Autodesk Fusion 360 part; units mm, degrees
sketch "Sketch1" plane through (0, 0, 0) normal (0, 1, 0) x (1, 0, 0)
  line L0 (7, -3.5) -> (-7, -3.5)
  line L1 (-7, -3.5) -> (-7, 3.5)
  line L2 (-7, 3.5) -> (7, 3.5)
  line L3 (7, 3.5) -> (7, -3.5)
  line L4 (7, -3.5) -> (-7, 3.5) construction
  line L5 (-7, -3.5) -> (7, 3.5) construction
  circle A0 centre (-6, 0) radius 0.5
  circle A1 centre (-1, 0) radius 0.5
  circle A2 centre (1, 0) radius 0.5
  circle A3 centre (6, 0) radius 0.5
  dimension "d3" = 14
  dimension "d4" = 7
  dimension "d7" = 1
  dimension "d8" = 1
  dimension "d9" = 1
  dimension "d10" = 1
sketch "Sketch2" plane through (0, 0, 0) normal (0, -1, 0) x (1, 0, 0)
  circle A0 centre (-1, 0) radius 0.5
  circle A1 centre (1, 0) radius 0.5
  circle A2 centre (6, 0) radius 0.5
  circle A3 centre (-6, 0) radius 0.5
  line L0 (-7, -3.5) -> (7, -3.5)
  line L1 (7, -3.5) -> (7, 3.5)
  line L2 (7, 3.5) -> (-7, 3.5)
  line L3 (-7, 3.5) -> (-7, -3.5)
  line L4 (-6, 2.5) -> (-6, -2.5)
  line L5 (6, -2.5) -> (6, 2.5)
  line L6 (6, -2.5) -> (1, -2.5)
  line L7 (1, -2.5) -> (1, 2.5)
  line L8 (1, 2.5) -> (6, 2.5)
  line L9 (-6, -2.5) -> (-6, 2.5)
  line L10 (-6, 2.5) -> (-1, 2.5)
  line L11 (-1, 2.5) -> (-1, -2.5)
  line L12 (-1, -2.5) -> (-6, -2.5)
sketch "Sketch3" plane through (0, 0, 0) normal (0, -1, 0) x (1, 0, 0)
sketch "Sketch4" plane through (0, 0, 0) normal (0, 1, 0) x (1, 0, 0)
  line L0 (-8, -5) -> (8, -5)
  line L1 (8, -5) -> (8, 5)
  line L2 (8, 5) -> (-8, 5)
  line L3 (-8, 5) -> (-8, -5)
  line L4 (-8, -5) -> (8, 5) construction
  line L5 (8, -5) -> (-8, 5) construction
  line L6 (-1, 0) -> (-1, -3)
  line L7 (-1, -3) -> (-7, -3)
  line L8 (-7, -3) -> (-7, 3)
  line L9 (-7, 3) -> (-1, 3)
  line L10 (-1, 3) -> (-1, 0)
  line L11 (1, 3) -> (1, -3)
  line L12 (1, -3) -> (7, -3)
  line L13 (7, -3) -> (7, 3)
  line L14 (7, 3) -> (1, 3)
  dimension "d16" = 16
  dimension "d17" = 10
sketch "Sketch5" plane through (0, 0, 0) normal (0, -1, 0) x (1, 0, 0)
  line L0 (-8, 5) -> (-8, -5)
  line L1 (-8, -5) -> (8, -5)
  line L2 (8, -5) -> (8, 5)
  line L3 (8, 5) -> (-8, 5)
  line L4 (-1, -3) -> (-1, 3)
  line L5 (-1, 3) -> (-7, 3)
  line L6 (-7, 3) -> (-7, -3)
  line L7 (-7, -3) -> (-1, -3)
  line L8 (1, -3) -> (1, 3)
  line L9 (1, 3) -> (7, 3)
  line L10 (7, 3) -> (7, -3)
  line L11 (7, -3) -> (1, -3)
sketch "Sketch6" plane through (0, 0, 0) normal (0, -1, 0) x (1, 0, 0)
  line L0 (-1, 3) -> (-1, -3)
  line L1 (-1, -3) -> (-7, -3)
  line L2 (-7, -3) -> (-7, 3)
  line L3 (-7, 3) -> (-1, 3)
  line L4 (1, 3) -> (7, 3)
  line L5 (7, 3) -> (7, -3)
  line L6 (7, -3) -> (1, -3)
  line L7 (1, -3) -> (1, 3)
  line L8 (-8, 5) -> (-8, -5)
  line L9 (-8, -5) -> (8, -5)
  line L10 (8, -5) -> (8, 5)
  line L11 (8, 5) -> (-8, 5)
  circle A0 centre (-7, 0) radius 0.25
  circle A1 centre (-1, 0) radius 0.25
  circle A2 centre (1, 0) radius 0.25
  circle A3 centre (7, 0) radius 0.25
  dimension "d23" = 0.5
  dimension "d24" = 0.5
  dimension "d25" = 0.5
  dimension "d26" = 0.5
sketch "Sketch7" plane through (0, 4, 0) normal (0, 1, 0) x (-1, 0, 0)
  circle A0 centre (1, 0) radius 0.25
  circle A1 centre (-1, 0) radius 0.25
  circle A2 centre (7, 0) radius 0.25
  circle A3 centre (-7, 0) radius 0.25
  line L0 (8, -5) -> (8, 5)
  line L1 (8, 5) -> (-8, 5)
  line L2 (-8, 5) -> (-8, -5)
  line L3 (-8, -5) -> (8, -5)
  line L4 (-10, -7) -> (10, -7)
  line L5 (10, -7) -> (10, 7)
  line L6 (10, 7) -> (-10, 7)
  line L7 (-10, 7) -> (-10, -7)
  circle A4 centre (-7, 0) radius 0.25
  circle A5 centre (-1, 0) radius 0.25
  circle A6 centre (1, 0) radius 0.25
  circle A7 centre (7, 0) radius 0.25
  dimension "d29" = 2
sketch "Sketch8" plane through (0, 0, 0) normal (0, -1, 0) x (1, 0, 0)
  line L0 (-8, 5) -> (-8, -5)
  line L1 (-8, -5) -> (8, -5)
  line L2 (8, -5) -> (8, 5)
  line L3 (8, 5) -> (-8, 5)
  arc A0 (1, 0.25) -> (1, -0.25) centre (1, 0) ccw
  line L4 (1, 0.25) -> (1, 3)
  line L5 (1, 3) -> (7, 3)
  line L6 (7, 3) -> (7, 0.25)
  arc A1 (7, -0.25) -> (7, 0.25) centre (7, 0) ccw
  line L7 (7, -0.25) -> (7, -3)
  line L8 (7, -3) -> (1, -3)
  line L9 (1, -3) -> (1, -0.25)
  arc A2 (-1, -0.25) -> (-1, 0.25) centre (-1, 0) ccw
  line L10 (-1, -0.25) -> (-1, -3)
  line L11 (-1, -3) -> (-7, -3)
  line L12 (-7, -3) -> (-7, -0.25)
  arc A3 (-7, 0.25) -> (-7, -0.25) centre (-7, 0) ccw
  line L13 (-7, 0.25) -> (-7, 3)
  line L14 (-7, 3) -> (-1, 3)
  line L15 (-1, 3) -> (-1, 0.25)
  circle A4 centre (-6.5, 4) radius 0.5
  circle A5 centre (-6.5, -4) radius 0.5
  circle A6 centre (6.5, -4) radius 0.5
  circle A7 centre (6.5, 4) radius 0.5
ref_plane "WorkPlane1" through (0, -6, 0) normal (0, -1, 0) x (-1, 0, 0)
sketch "Sketch11" plane through (0, 0, 0) normal (0, -1, 0) x (1, 0, 0)
sketch "Sketch12" plane through (0, 4, 0) normal (0, 1, 0) x (-1, 0, 0)
  circle A0 centre (1, 0) radius 0.25
  circle A1 centre (-1, 0) radius 0.25
  circle A2 centre (7, 0) radius 0.25
  circle A3 centre (-7, 0) radius 0.25
  line L0 (-11, -8) -> (11, -8)
  line L1 (11, -8) -> (11, 8)
  line L2 (11, 8) -> (-11, 8)
  line L3 (-11, 8) -> (-11, -8)
sketch "Sketch13" plane through (0, 0, 0) normal (0, -1, 0) x (1, 0, 0)
sketch "Sketch14" plane through (0, 0, 0) normal (0, -1, 0) x (1, 0, 0)
sketch "Sketch15" plane through (0, 0, 0) normal (0, 1, 0) x (1, 0, 0)
  line L0 (8, -5) -> (-8, -5)
  line L1 (-8, -5) -> (-8, 5)
  line L2 (-8, 5) -> (8, 5)
  line L3 (8, 5) -> (8, -5)
  line L4 (8, -5) -> (-8, 5) construction
  line L5 (-8, -5) -> (8, 5) construction
  dimension "d43" = 16
  dimension "d44" = 10
extrude "Extrude9" add sketch "Sketch15" along normal blind 5
sketch "Sketch16" plane through (0, 0, 0) normal (0, -1, 0) x (1, 0, 0)
  line L0 (-8, -5) -> (8, -5)
  line L1 (8, -5) -> (8, 5)
  line L2 (8, 5) -> (-8, 5)
  line L3 (-8, 5) -> (-8, -5)
  line L4 (7, 3) -> (1, 3)
  line L5 (1, 3) -> (1, -3)
  line L6 (1, -3) -> (7, -3)
  line L7 (7, -3) -> (7, 3)
  line L8 (7, 3) -> (1, -3) construction
  line L9 (1, 3) -> (7, -3) construction
  line L10 (-1, 0) -> (-4, 0)
  line L11 (-1, 0) -> (-1, 3)
  line L12 (-1, 0) -> (-1, -3)
  line L13 (-1, -3) -> (-7, -3)
  line L14 (-7, -3) -> (-7, 3)
  line L15 (-7, 3) -> (-1, 3)
  point P0 (4, 0)
  dimension "d48" = 6
  dimension "d49" = 6
  dimension "d50" = 1
  dimension "d51" = 3
  dimension "d52" = 3
  dimension "d53" = 6
  dimension "d54" = 6
extrude "Extrude10" cut sketch "Sketch16" against normal blind 3 contours L4 L5 L6 L7 | L11 L12 L13 L14 L15
sketch "Sketch17" plane through (0, 0, 0) normal (0, -1, 0) x (1, 0, 0)
  line L0 (-7, 3) -> (-1, 3)
  line L1 (-1, 3) -> (-1, -3)
  line L2 (-1, -3) -> (-7, -3)
  line L3 (-7, -3) -> (-7, 3)
  line L4 (1, 3) -> (7, 3)
  line L5 (7, 3) -> (7, -3)
  line L6 (7, -3) -> (1, -3)
  line L7 (1, -3) -> (1, 3)
  line L8 (-8, -5) -> (8, -5)
  line L9 (8, -5) -> (8, 5)
  line L10 (8, 5) -> (-8, 5)
  line L11 (-8, 5) -> (-8, -5)
  line L12 (-10, -7) -> (10, -7)
  line L13 (10, -7) -> (10, 7)
  line L14 (10, 7) -> (-10, 7)
  line L15 (-10, 7) -> (-10, -7)
  dimension "d57" = 2
extrude "Extrude11" add sketch "Sketch17" along normal blind 3 and the other way blind 1 contours L12 L13 L14 L15
sketch "Sketch18" plane through (0, 0, 0) normal (0, -1, 0) x (1, 0, 0)
  line L0 (-7, 3) -> (-1, 3)
  line L1 (-1, 3) -> (-1, -3)
  line L2 (-1, -3) -> (-7, -3)
  line L3 (-7, -3) -> (-7, 3)
  line L4 (1, 3) -> (7, 3)
  line L5 (7, 3) -> (7, -3)
  line L6 (7, -3) -> (1, -3)
  line L7 (1, -3) -> (1, 3)
  line L8 (-8, -5) -> (8, -5)
  line L9 (8, -5) -> (8, 5)
  line L10 (8, 5) -> (-8, 5)
  line L11 (-8, 5) -> (-8, -5)
  circle A0 centre (1, 0) radius 0.5
  circle A1 centre (7, 0) radius 0.5
  circle A2 centre (-1, 0) radius 0.5
  circle A3 centre (-7, 0) radius 0.5
  dimension "d62" = 1
  dimension "d63" = 1
  dimension "d64" = 1
  dimension "d65" = 1
extrude "Extrude12" cut sketch "Sketch18" against normal blind 5 contours L3 A3 | L3 A3 | L1 A2 | L1 A2 | L7 A0 | L7 A0 | L5 A1 | L5 A1
sketch "Sketch19" plane through (0, 0, 0) normal (0, -1, 0) x (1, 0, 0)
  line L0 (-8, -5) -> (8, -5)
  line L1 (8, 5) -> (-8, 5)
  line L2 (-8, 5) -> (-8, -5)
  arc A0 (1, 0.5) -> (1, -0.5) centre (1, 0) ccw
  arc A1 (7, -0.5) -> (7, 0.5) centre (7, 0) ccw
  line L3 (7, -3) -> (1, -3)
  line L4 (1, -3) -> (1, -0.5)
  arc A2 (-1, -0.5) -> (-1, 0.5) centre (-1, 0) ccw
  line L5 (-1, -0.5) -> (-1, -3)
  line L6 (-1, -3) -> (-7, -3)
  line L7 (-7, -3) -> (-7, -0.5)
  arc A3 (-7, 0.5) -> (-7, -0.5) centre (-7, 0) ccw
  line L8 (-7, 0.5) -> (-7, 3)
  line L9 (-7, 3) -> (-1, 3)
  line L10 (-8, 5) -> (8, 5)
  line L11 (8, 5) -> (8, -5)
  line L12 (8, -5) -> (-8, -5)
  line L13 (-8, -5) -> (-8, 5)
sketch "Sketch20" plane through (0, -10, 0) normal (0, 1, 0) x (-1, 0, 0)
  line L0 (-8, -5) -> (8, -5)
  line L1 (8, -5) -> (8, 5)
  line L2 (8, 5) -> (-8, 5)
  line L3 (-8, 5) -> (-8, -5)
  line L4 (-7, -4) -> (7, -4)
  line L5 (7, -4) -> (7, 4)
  line L6 (7, 4) -> (-7, 4)
  line L7 (-7, 4) -> (-7, -4)
  dimension "d73" = -1
sketch "Sketch21" plane through (0, -13, 0) normal (0, -1, 0) x (1, 0, 0)
  line L0 (-8, -5) -> (8, -5)
  line L1 (8, -5) -> (8, 5)
  line L2 (8, 5) -> (-8, 5)
  line L3 (-8, 5) -> (-8, -5)
  circle A0 centre (-4, 0) radius 2
  circle A1 centre (4, 0) radius 2
Geometry check sheet. Reference: the model listing, model coordinates, mm. A direction names the side the tool comes from. Round coordinates to 2 decimals unless told otherwise and drop trailing zeros. Loops run counter-clockwise (first coordinate to the right, second up) from the corner with the lowest first, then second, coordinate; pieces in that order, holes last. Notation, with made-up numbers: (48.25, 5) - (91.25, 5) arc R24 ccw to (91.25, 28) - close; hole circle Ø1 at (10.5, 55.25). An arc over 180 degrees is marked (long way). One line per question, with ' | ' between items. Start each with the question number.
1. Cross-section at A-A on y = 2.75. Record the cut outline in (x, z).
2. Draft check along X on faces 1 (the face through (10, -1, 0)), 2 (the face through (0, 1, -6)), 3 (the face through (1, 1, 2)). Enter one of: released by +X, released by -X, zero draft, split by the parting line, or undercut.
3. Cross-section at D-D on z = -2.75. Record the cut outline in (x, y).
4. Tool access check on faces 4 (the face through (-7, 1, 2)), 5 (the face through (0, -1, 7)). Record the directions out of +Z, -Z, +X, -X, +Y, -Y that give a thin tool (end or side, any length) a straight path to the whole face; none if there is none.
5. Depth check by flat-ended pin: pin 1 (5 mm diameter, centred on x = -4, z = 2, fed in from -Y); pin 2 (0.9 mm diameter, centred on x = 5, y = 1.5, fed in from -Z); pin 3 (3 mm diameter, centred on y = 2, z = 2, fed in from -X); pin 4 (1.2 mm diameter, centred on y = 2, z = -1.5, fed in from -X). Enter the tip coordinate at first touch or a pass-through.
6. Cross-section at B-B on z = 0. Record the cut outline in (x, y), then the cut area to 3 significant figures.
7. Cross-section at C-C on x = -7.75. Record the cut outline in (y, z), then the cut area to 3 significant figures.
8. Scan lines: line 1 (X direction, y = 1.55, z = 0); line 2 (X direction, y = 2.25, z = 0.75); line 3 (X direction, y = 3.45, z = 0). Record each from-to range of solid material in increasing order. Write a range as [from, to].
Taken from the geometry:
1) outline: (-8, -5) - (8, -5) - (8, 5) - (-8, 5) - close; hole (-7, -3) - (-1, -3) - (-1, -0.5) arc R0.5 ccw to (-1, 0.5) - (-1, 3) - (-7, 3) - (-7, 0.5) arc R0.5 ccw to (-7, -0.5) - close; hole (1, -3) - (7, -3) - (7, -0.5) arc R0.5 ccw to (7, 0.5) - (7, 3) - (1, 3) - (1, 0.5) arc R0.5 ccw to (1, -0.5) - close
2) face 1: released by +X | face 2: zero draft | face 3: undercut
3) outline: (-10, -3) - (-8, -3) - (-8, 0) - (-7, 0) - (-7, 3) - (-1, 3) - (-1, 0) - (1, 0) - (1, 3) - (7, 3) - (7, 0) - (8, 0) - (8, -3) - (10, -3) - (10, 1) - (8, 1) - (8, 5) - (-8, 5) - (-8, 1) - (-10, 1) - close
4) face 4: -Y | face 5: +Z, +X, -X, +Y, -Y
5) pin 1: y = 0 | pin 2: z = -5 | pin 3: x = -10 | pin 4: x = -8
6) outline: (-10, -3) - (-8, -3) - (-8, 0) - (-7.5, 0) - (-7.5, 5) - (-8, 5) - (-8, 1) - (-10, 1) - close; (-6.5, 3) - (-1.5, 3) - (-1.5, 5) - (-6.5, 5) - close; (-0.5, 0) - (0.5, 0) - (0.5, 5) - (-0.5, 5) - close; (1.5, 3) - (6.5, 3) - (6.5, 5) - (1.5, 5) - close; (7.5, 0) - (8, 0) - (8, -3) - (10, -3) - (10, 1) - (8, 1) - (8, 5) - (7.5, 5) - close | area: 46.0 mm²
7) outline: (-3, -7) - (1, -7) - (1, -5) - (5, -5) - (5, 5) - (1, 5) - (1, 7) - (-3, 7) - (-3, 5) - (0, 5) - (0, -5) - (-3, -5) - close | area: 66.0 mm²
8) line 1: [-8, -7.5], [-0.5, 0.5], [7.5, 8] | line 2: [-8, -7], [-1, 1], [7, 8] | line 3: [-8, -7.5], [-6.5, -1.5], [-0.5, 0.5], [1.5, 6.5], [7.5, 8]
